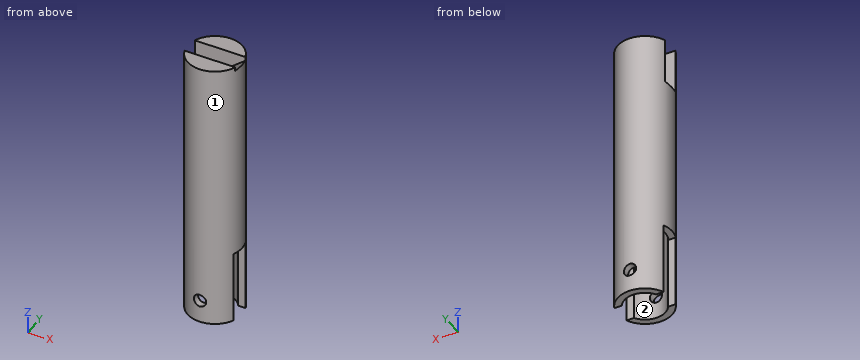
```python
from build123d import *

# Parameters (mm, degrees)
F0_R          = 2.4
F1_DEPTH      = 24
F2_R          = 1.8
F3_DEPTH      = 10
F5_DEPTH      = 25
F5_DEPTH_BACK = 25
F7_DEPTH      = 0.8
F7_DEPTH_BACK = 0.8
F8_R          = 0.55
F9_DEPTH      = 2.401
F9_DEPTH_BACK = 2.401


with BuildPart() as f1:
    # F0 (on Top) → F1 (new body)
    with BuildSketch(Plane.XY):
        Circle(F0_R)
    extrude(amount=F1_DEPTH)

    # F2 (on face) → F3 (cut)
    with BuildSketch(Plane(origin=(0, 0, 0), x_dir=(1, 0, 0), z_dir=(0, 0, -1))):
        Circle(F2_R)
    extrude(amount=-F3_DEPTH, mode=Mode.SUBTRACT)

    # F4 (on Right) → F5 (cut, two sides)
    with BuildSketch(Plane.YZ) as f5_sk:
        Polygon((-0.95, 0), (0.95, 0), (0.95, 6.3333333333), (0, 6.3333333333), (-0.95, 6.3333333333), align=None)
    extrude(amount=-F5_DEPTH, mode=Mode.SUBTRACT)
    extrude(f5_sk.sketch, amount=F5_DEPTH_BACK, mode=Mode.SUBTRACT)

    # F6 (on Front) → F7 (cut, two sides)
    with BuildSketch(Plane.XZ) as f7_sk:
        Polygon((-2.4, 24), (-2.4946786115, 24), (-2.4946786115, 19.9), (2.7053213885, 24), (2.4, 24), align=None)
    extrude(amount=F7_DEPTH, mode=Mode.SUBTRACT)
    extrude(f7_sk.sketch, amount=-F7_DEPTH_BACK, mode=Mode.SUBTRACT)

    # F8 (on Front) → F9 (cut, two sides)
    with BuildSketch(Plane.XZ) as f9_sk:
        with Locations((0, 2)):
            Circle(F8_R)
    extrude(amount=-F9_DEPTH, mode=Mode.SUBTRACT)
    extrude(f9_sk.sketch, amount=F9_DEPTH_BACK, mode=Mode.SUBTRACT)


solid = f1.part
```
Check sheet for the modelled part. Datum: model origin and axes. Units: mm. Face numbers are marked on the shaded views. Give positions to 0.01 mm unless a question says otherwise; leave off trailing zeros. Order: outer loops, then holes, each group sorted by start corner. A loop starts at its lowest first (then second) coordinate and runs counter-clockwise, first axis right, second up. Notation, with made-up numbers: (6, 85.5) -> (34, 85.5) arc R21 ccw to (34, 110.5) -> close; hole circle Ø5 at (38, -37). An arc over 180 degrees is marked (long way). Use CSV: the item, a comma, the result in double quotes. Start each with the question number.
1) Sectioned sample at C-C, the plane y = 0. Record the boundary of the cut face in (x, z), plus the area to 3 significant figures.
2) Material ranges on line 1 (Z direction, x = 0, y = -2); line 2 (X direction, y = -1.85, z = 2); line 3 (X direction, y = 0, z = 6.5), recorded low to high. Write a range as from..to.
3) Go/stop test with flat-tipped pins: P1, Ø1, axis at x = 2, y = 0, coming from the -Z side; P2, Ø0.7, axis at x = -2, z = 4.5, coming from the -Y side; P3, Ø1, axis at y = -1.5, z = 13.5, coming from the -X side. Record where each tip stops, or that it passes through.
4) Sectioned sample at D-D, the plane z = 2. Record the boundary of the cut face in (x, y).
5) Sectioned sample at B-B, the plane x = 0.1. Record the boundary of the cut face in (y, z).
6) Sectioned sample at A-A, the plane z = 4.5. Record the boundary of the cut face in (x, y), plus the area to 3 significant figures.
7) Mould release check, pull along X, two halves, no side actions. Record for the marked faces 1 and 2: released by +X, released by -X, zero draft, split by the parting line, or undercut.
Recorded:
1,outline,"(-2.4, 6.33) -> (-1.8, 6.33) -> (-1.8, 10) -> (1.8, 10) -> (1.8, 6.33) -> (2.4, 6.33) -> (2.4, 23.76) -> (-2.4, 19.97) -> close"
1,area,"61.4 mm2"
2,line 1,"0..1.45, 2.55..24"
2,line 2,"-1.53..-0.55, 0.55..1.53"
2,line 3,"-2.4..-1.8, 1.8..2.4"
3,P1,"z = 6.33"
3,P2,"y = -1.74"
3,P3,"x = -2.18"
4,outline,"(-2.2, -0.95) arc R2.4 ccw to (-0.55, -2.34) -> (-0.55, -1.71) arc R1.8 cw to (-1.53, -0.95) -> close; (-2.2, 0.95) -> (-1.53, 0.95) arc R1.8 cw to (-0.55, 1.71) -> (-0.55, 2.34) arc R2.4 ccw to start; (0.55, -2.34) arc R2.4 ccw to (2.2, -0.95) -> (1.53, -0.95) arc R1.8 cw to (0.55, -1.71) -> close; (0.55, 1.71) arc R1.8 cw to (1.53, 0.95) -> (2.2, 0.95) arc R2.4 ccw to (0.55, 2.34) -> close"
5,outline,"(-2.4, 0) -> (-1.8, 0) -> (-1.8, 1.46) -> (-2.4, 1.46) -> close; (-2.4, 2.54) -> (-1.8, 2.54) -> (-1.8, 10) -> (1.8, 10) -> (1.8, 2.54) -> (2.4, 2.54) -> (2.4, 24) -> (0.8, 24) -> (0.8, 21.95) -> (-0.8, 21.95) -> (-0.8, 24) -> (-2.4, 24) -> close; (1.8, 0) -> (2.4, 0) -> (2.4, 1.46) -> (1.8, 1.46) -> close"
6,outline,"(-2.2, -0.95) arc R2.4 ccw to (2.2, -0.95) -> (1.53, -0.95) arc R1.8 cw to (-1.53, -0.95) -> close; (-2.2, 0.95) -> (-1.53, 0.95) arc R1.8 cw to (1.53, 0.95) -> (2.2, 0.95) arc R2.4 ccw to start"
6,area,"5.55 mm2"
7,face 1,"split by the parting line"
7,face 2,"undercut"
